Geometry check sheet. Reference: the model listing, model coordinates, mm. Face numbers are marked on the shaded views. A direction names the side the tool comes from. Coordinates: 2 decimals unless noted, no trailing zeros.
from build123d import *

# Parameters (mm, degrees)
SKETCH1_W               = 101.6
SKETCH1_H               = 101.6
SKETCH1_R               = 38.394
SKETCH1_R_2             = 3.175
SKETCH1_R_3             = 11.8745
SKETCH1_R_4             = 4.1275
BOSS_EXTRUDE1_DEPTH     = 6.35
SKETCH2_W               = 101.6
SKETCH2_H               = 101.6
SKETCH2_R               = 38.227
BOSS_EXTRUDE2_DEPTH     = 15.875
BOSS_EXTRUDE3_DEPTH     = 3.81
SKETCH8_R               = 6.477
CUT_EXTRUDE1_DEPTH      = 10.16
CUT_EXTRUDE5_DEPTH      = 76.201267443
CIRPATTERN1_START       = 40.64
CIRPATTERN1_OUTLINE_R   = 6.477
CIRPATTERN1_DEPTH       = 10.16
CIRPATTERN1_START_2     = -50.8
CIRPATTERN1_2_OUTLINE_R = 6.477
CIRPATTERN1_2_DEPTH     = 10.16
CIRPATTERN1_3_OUTLINE_R = 6.477
CIRPATTERN1_3_DEPTH     = 10.16
CIRPATTERN1_4_OUTLINE_R = 6.477
CIRPATTERN1_4_DEPTH     = 10.16
CIRPATTERN1_5_OUTLINE_R = 6.477
CIRPATTERN1_5_DEPTH     = 10.16
SKETCH13_R              = 2.54
CUT_EXTRUDE4_DEPTH      = 17.272
CIRPATTERN4_START       = 38.142521171
CIRPATTERN4_OUTLINE_R   = 2.54
CIRPATTERN4_DEPTH       = 2.497478829
CIRPATTERN4_START_2     = -40.64
CIRPATTERN4_2_OUTLINE_R = 2.54
CIRPATTERN4_2_DEPTH     = 81.28
CIRPATTERN4_3_OUTLINE_R = 2.54
CIRPATTERN4_3_DEPTH     = 2.497478829
CIRPATTERN4_4_OUTLINE_R = 2.54
CIRPATTERN4_4_DEPTH     = 2.497478829
SKETCH12_R              = 2.54
CUT_EXTRUDE3_DEPTH      = 74.575101958
FILLET1_R               = 12.7
CHAMFER1_SIZE           = 2.54
CHAMFER2_SIZE           = 0.635
CHAMFER3_SIZE           = 0.635


# Read off the part's stored shape, not the designer's step: Boss-Extrude3, CirPattern1, CirPattern4
with BuildPart() as part:
    # Sketch1 → Boss-Extrude1 (new body)
    # profile 1 of 9: a face of its own
    with BuildSketch(Plane(origin=(0, 0, 0), x_dir=(1, 0, 0), z_dir=(0, 1, 0))):
        Rectangle(SKETCH1_W, SKETCH1_H)
        Circle(SKETCH1_R, mode=Mode.SUBTRACT)
    # profile 2 of 9: a face of its own
    with BuildSketch(Plane(origin=(0, 0, 0), x_dir=(1, 0, 0), z_dir=(0, 1, 0))):
        Circle(SKETCH1_R)
        with Locations((0, 30.226)):
            Circle(SKETCH1_R_2, mode=Mode.SUBTRACT)
        with Locations((12.7, 20.066)):
            Circle(SKETCH1_R_3, mode=Mode.SUBTRACT)
        with Locations((0, 9.906)):
            Circle(SKETCH1_R_2, mode=Mode.SUBTRACT)
        with Locations((0, -14.605)):
            Circle(SKETCH1_R_4, mode=Mode.SUBTRACT)
        with Locations((-12.7, 20.066)):
            Circle(SKETCH1_R_3, mode=Mode.SUBTRACT)
        with Locations((25.4, 2.6162)):
            Circle(SKETCH1_R_2, mode=Mode.SUBTRACT)
        with Locations((-25.4, 2.6162)):
            Circle(SKETCH1_R_2, mode=Mode.SUBTRACT)
    # profile 3 of 9: a face of its own
    with BuildSketch(Plane(origin=(0, 0, 0), x_dir=(1, 0, 0), z_dir=(0, 1, 0))):
        with Locations((-25.4, 2.6162)):
            Circle(SKETCH1_R_2)
    # profile 4 of 9: a face of its own
    with BuildSketch(Plane(origin=(0, 0, 0), x_dir=(1, 0, 0), z_dir=(0, 1, 0))):
        with Locations((0, 9.906)):
            Circle(SKETCH1_R_2)
    # profile 5 of 9: a face of its own
    with BuildSketch(Plane(origin=(0, 0, 0), x_dir=(1, 0, 0), z_dir=(0, 1, 0))):
        with Locations((0, 30.226)):
            Circle(SKETCH1_R_2)
    # profile 6 of 9: a face of its own
    with BuildSketch(Plane(origin=(0, 0, 0), x_dir=(1, 0, 0), z_dir=(0, 1, 0))):
        with Locations((12.7, 20.066)):
            Circle(SKETCH1_R_3)
    # profile 7 of 9: a face of its own
    with BuildSketch(Plane(origin=(0, 0, 0), x_dir=(1, 0, 0), z_dir=(0, 1, 0))):
        with Locations((-12.7, 20.066)):
            Circle(SKETCH1_R_3)
    # profile 8 of 9: a face of its own
    with BuildSketch(Plane(origin=(0, 0, 0), x_dir=(1, 0, 0), z_dir=(0, 1, 0))):
        with Locations((0, -14.605)):
            Circle(SKETCH1_R_4)
    # profile 9 of 9: a face of its own
    with BuildSketch(Plane(origin=(0, 0, 0), x_dir=(1, 0, 0), z_dir=(0, 1, 0))):
        with Locations((25.4, 2.6162)):
            Circle(SKETCH1_R_2)
    extrude(amount=BOSS_EXTRUDE1_DEPTH)

    # Sketch2 → Boss-Extrude2 (add)
    with BuildSketch(Plane(origin=(0, 6.35, 0), x_dir=(1, 0, 0), z_dir=(0, 1, 0))):
        Rectangle(SKETCH2_W, SKETCH2_H)
        with Locations(Location((0, 0, 0), (0, 0, 270))):
            Circle(SKETCH2_R, mode=Mode.SUBTRACT)
    extrude(amount=BOSS_EXTRUDE2_DEPTH)

    # Boss-Extrude3 outline → Boss-Extrude3 (add)
    with BuildSketch(Plane(origin=(0, 6.35, 0), x_dir=(1, 0, 0), z_dir=(0, 1, 0))):
        with BuildLine():
            ThreePointArc((-24.172458524, 12.000725193), (-5.035808562, 5.942254103), (-7.873448726, 25.813445361))
            ThreePointArc((-7.873448726, 25.813445361), (-17.448004255, 20.58864502), (-24.172458524, 12.000725193))
        make_face()
        with BuildLine():
            ThreePointArc((24.172458524, 12.000725193), (17.448004255, 20.58864502), (7.873448726, 25.813445361))
            ThreePointArc((7.873448726, 25.813445361), (5.035808562, 5.942254103), (24.172458524, 12.000725193))
        make_face()
    extrude(amount=BOSS_EXTRUDE3_DEPTH)

    # Sketch8 → Cut-Extrude1 (cut)
    with BuildSketch(Plane(origin=(0, 0, -50.8), x_dir=(-1, 0, 0), z_dir=(0, 0, -1))):
        with Locations((0, 11.1125)):
            Circle(SKETCH8_R)
    extrude(amount=-CUT_EXTRUDE1_DEPTH, mode=Mode.SUBTRACT)

    # Sketch15 → Cut-Extrude5 (cut, through all)
    with BuildSketch(Plane(origin=(0, 22.225, 0), x_dir=(1, 0, 0), z_dir=(0, 1, 0))):
        Polygon((-50.8, 13.611818976), (-29.329393675, 50.8), (-50.8, 50.8), align=None)
        Polygon((-58.65878735, 0), (-50.8, 13.611818976), (-50.8, 50.8), (-58.65878735, 50.8), align=None)
        Polygon((-50.8, -13.611818976), (-50.8, 13.611818976), (-58.65878735, 0), align=None)
        Polygon((-50.8, -13.611818976), (-58.65878735, 0), (-58.65878735, -50.8), (-50.8, -50.8), align=None)
        Polygon((-29.329393675, -50.8), (-50.8, -13.611818976), (-50.8, -50.8), align=None)
        Polygon((50.8, -50.8), (50.8, -13.611818976), (29.329393675, -50.8), align=None)
        Polygon((58.65878735, -50.8), (58.65878735, 0), (50.8, -13.611818976), (50.8, -50.8), align=None)
        Polygon((58.65878735, 0), (50.8, 13.611818976), (50.8, -13.611818976), align=None)
        Polygon((50.8, 50.8), (50.8, 13.611818976), (58.65878735, 0), (58.65878735, 50.8), align=None)
        Polygon((50.8, 50.8), (29.329393675, 50.8), (50.8, 13.611818976), align=None)
    extrude(amount=-CUT_EXTRUDE5_DEPTH, mode=Mode.SUBTRACT)

    # CirPattern1 outline → CirPattern1 (cut)
    with BuildSketch(Plane.XY.offset(CIRPATTERN1_START)):
        with Locations((0, 11.1125)):
            Circle(CIRPATTERN1_OUTLINE_R)
    extrude(amount=CIRPATTERN1_DEPTH, mode=Mode.SUBTRACT)

    # CirPattern1 2 outline → CirPattern1 2 (cut)
    with BuildSketch(Plane(origin=(0, 0, 0), x_dir=(0.49999999999999195, 0, 0.8660254037844434), z_dir=(0.8660254037844433, 0, -0.4999999999999921)).offset(CIRPATTERN1_START_2)):
        with Locations((0, -11.1125)):
            Circle(CIRPATTERN1_2_OUTLINE_R)
    extrude(amount=CIRPATTERN1_2_DEPTH, mode=Mode.SUBTRACT)

    # CirPattern1 3 outline → CirPattern1 3 (cut)
    with BuildSketch(Plane(origin=(0, 0, 0), x_dir=(0.500000000000004, 0, -0.8660254037844363), z_dir=(0.8660254037844363, 0, 0.5000000000000042)).offset(CIRPATTERN1_START)):
        with Locations((0, 11.1125)):
            Circle(CIRPATTERN1_3_OUTLINE_R)
    extrude(amount=CIRPATTERN1_3_DEPTH, mode=Mode.SUBTRACT)

    # CirPattern1 4 outline → CirPattern1 4 (cut)
    with BuildSketch(Plane.YZ.offset(CIRPATTERN1_START_2)):
        with Locations((11.1125, 0)):
            Circle(CIRPATTERN1_4_OUTLINE_R)
    extrude(amount=CIRPATTERN1_4_DEPTH, mode=Mode.SUBTRACT)

    # CirPattern1 5 outline → CirPattern1 5 (cut)
    with BuildSketch(Plane.YZ.offset(CIRPATTERN1_START)):
        with Locations((11.1125, 0)):
            Circle(CIRPATTERN1_5_OUTLINE_R)
    extrude(amount=CIRPATTERN1_5_DEPTH, mode=Mode.SUBTRACT)

    # Sketch13 → Cut-Extrude4 (cut)
    with BuildSketch(Plane(origin=(0, 0, -50.8), x_dir=(-1, 0, 0), z_dir=(0, 0, -1))):
        with Locations((0, 11.1125)):
            Circle(SKETCH13_R)
    extrude(amount=-CUT_EXTRUDE4_DEPTH, mode=Mode.SUBTRACT)

    # CirPattern4 outline → CirPattern4 (cut)
    with BuildSketch(Plane.XY.offset(CIRPATTERN4_START)):
        with Locations((0, 11.1125)):
            Circle(CIRPATTERN4_OUTLINE_R)
    extrude(amount=CIRPATTERN4_DEPTH, mode=Mode.SUBTRACT)

    # CirPattern4 2 outline → CirPattern4 2 (cut)
    with BuildSketch(Plane.YZ.offset(CIRPATTERN4_START_2)):
        with Locations((11.1125, 0)):
            Circle(CIRPATTERN4_2_OUTLINE_R)
    extrude(amount=CIRPATTERN4_2_DEPTH, mode=Mode.SUBTRACT)

    # CirPattern4 3 outline → CirPattern4 3 (cut)
    with BuildSketch(Plane(origin=(0, 0, 0), x_dir=(0.49999999999999195, 0, -0.8660254037844434), z_dir=(0.8660254037844433, 0, 0.4999999999999921)).offset(CIRPATTERN4_START)):
        with Locations((0, 11.1125)):
            Circle(CIRPATTERN4_3_OUTLINE_R)
    extrude(amount=CIRPATTERN4_3_DEPTH, mode=Mode.SUBTRACT)

    # CirPattern4 4 outline → CirPattern4 4 (cut)
    with BuildSketch(Plane(origin=(0, 0, 0), x_dir=(0.500000000000004, 0, 0.8660254037844363), z_dir=(0.8660254037844363, 0, -0.5000000000000042)).offset(CIRPATTERN4_START_2)):
        with Locations((0, -11.1125)):
            Circle(CIRPATTERN4_4_OUTLINE_R)
    extrude(amount=CIRPATTERN4_4_DEPTH, mode=Mode.SUBTRACT)

    # Sketch12 → Cut-Extrude3 (cut, through all)
    with BuildSketch(Plane(origin=(0, 6.35, 0), x_dir=(1, 0, 0), z_dir=(0, 1, 0))):
        with Locations(Location((-30.913047265, -9.296856721, 0), (0, 0, 270))):
            Circle(SKETCH12_R)
        with Locations(Location((31.335909349, -9.296856721, 0), (0, 0, 270))):
            Circle(SKETCH12_R)
        with Locations(Location((0, -32.997501828, 0), (0, 0, 270))):
            Circle(SKETCH12_R)
        with Locations(Location((0, 31.87799304, 0), (0, 0, 270))):
            Circle(SKETCH12_R)
    extrude(amount=-CUT_EXTRUDE3_DEPTH, mode=Mode.SUBTRACT)

    # Fillet1
    fillet1_edges = [part.edges().sort_by_distance(p)[0] for p in [
        (-29.329393675, 11.1125, -50.8),
        (-50.8, 11.1125, -13.611818976),
        (-50.8, 11.1125, 13.611818976),
        (-29.329393675, 11.1125, 50.8),
        (29.329393675, 11.1125, -50.8),
        (29.329393675, 11.1125, 50.8),
        (50.8, 11.1125, 13.611818976),
        (50.8, 11.1125, -13.611818976),
    ]]
    fillet(fillet1_edges, radius=FILLET1_R)

    # Chamfer1
    chamfer1_edges = [part.edges().sort_by_distance(p)[0] for p in [
        (0, 22.225, -38.227),
    ]]
    chamfer(chamfer1_edges, length=CHAMFER1_SIZE)

    # Chamfer2
    chamfer2_edges = [part.edges().sort_by_distance(p)[0] for p in [
        (-5.035808562, 10.16, -5.942254103),
        (-17.448004255, 10.16, -20.58864502),
        (5.035808562, 10.16, -5.942254103),
        (17.448004255, 10.16, -20.58864502),
    ]]
    chamfer(chamfer2_edges, length=CHAMFER2_SIZE)

    # Chamfer3
    chamfer3_edges = [part.edges().sort_by_distance(p)[0] for p in [
        (-41.047045256, 22.225, 30.504432116),
        (0, 22.225, -50.8),
        (-41.047045256, 22.225, -30.504432116),
        (-50.8, 22.225, 0),
        (0, 22.225, 50.8),
        (41.047045256, 22.225, 30.504432116),
        (50.8, 22.225, 0),
        (41.047045256, 22.225, -30.504432116),
        (28.347045256, 22.225, 49.098522628),
        (50.367257994, 22.225, 13.495866104),
        (50.367257994, 22.225, -13.495866104),
        (28.347045256, 22.225, -49.098522628),
        (-28.347045256, 22.225, -49.098522628),
        (-50.367257994, 22.225, -13.495866104),
        (-50.367257994, 22.225, 13.495866104),
        (-28.347045256, 22.225, 49.098522628),
    ]]
    chamfer(chamfer3_edges, length=CHAMFER3_SIZE)


solid = part.part
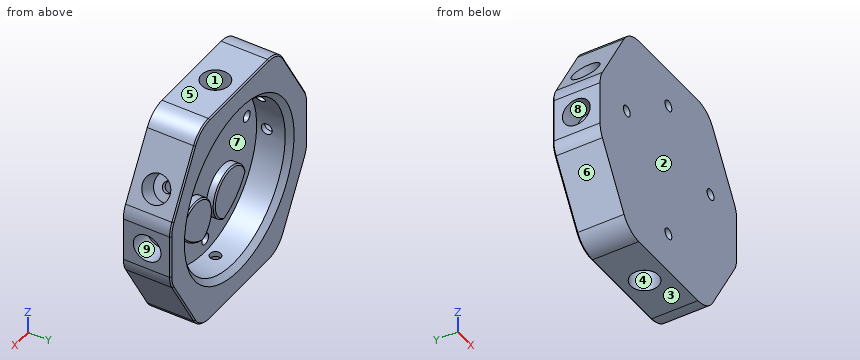
1. Thickness scan on line 1 along Z through (x, y) = (19.5, 8.5); line 2 along Z through (x, y) = (21, 9.25); line 3 along Z through (x, y) = (-26, 3.25). Record the ranges inside material, lowest first.
Computed values:
line 1: z = -50.8 to -32.88, -18.66 to -5.28, 32.88 to 50.8
line 2: z = -50.8 to -31.94, -16.95 to -6.52, 31.94 to 50.8
line 3: z = -50.15 to 50.15
2. Access from +Z, -Z, +X, -X, +Y, -Y to the whole of each face (thin tool, end or side, straight path). Record for the marked faces 5, 6, 7, 8 and 9.
Computed values:
face 5: +Z, +X, -X, +Y, -Y
face 6: -Z, -X, +Y, -Y
face 7: +Y
face 8: -X
face 9: +X
3. Gauge pin test, flat ends, axial feed: pin 1 Ø3 at (x, y) = (0, 11.11) entering from -Z; pin 2 Ø4 at (x, y) = (30, 13.5) entering from +Z; pin 3 Ø10 at (y, z) = (14.5, -16.5) entering from +X; pin 4 Ø6 at (y, z) = (16.5, -25.5) entering from +X. Record the tip position at first contact, or that the pin passes through.
Computed values:
pin 1: passes through
pin 2: stops at z = 49.29
pin 3: stops at x = 50.73
pin 4: stops at x = 45.67
4. Draft check along Y on the marked faces 1, 2, 3 and 4. Enter one of: released by +Y, released by -Y, zero draft, split by the parting line, or undercut.
Computed values:
face 1: undercut
face 2: released by -Y
face 3: zero draft
face 4: undercut
